Design review of the part built by this model. Coordinates are the model's own, in mm. Give positions to 0.01 mm unless a question says otherwise; leave off trailing zeros. Loops run counter-clockwise (first coordinate to the right, second up) from the corner with the lowest first, then second, coordinate; pieces in that order, holes last. Notation, with made-up numbers: M 57.25,-22.5 L 76.25,-22.5 A8 ccw 76.25,-15.5 Z; hole C 30,13 d4. An arc over 180 degrees is marked long. Use a Markdown table: item, result. Add a question column.
(1) Add section A-A, the plane y = 30. Give the boundary of the cut face in (x, z).
(2) Insertion check: pin 1 Ø3.5 at (x, y) = (115, 60) entering from +Z. The pin has a flat end and moves straight along its axis. Give the tip position at first contact, or say it passes through.
(3) For probe 1 along Y at (x, z) = (43, 0.75); probe 2 along X at (y, z) = (115, 0.9); probe 3 along X at (y, z) = (24.75, 0.8), list the stretches that pass through material, from the lowest coordinate up.
(4) Add section D-D, the plane x = 43. Give the boundary of the cut face in (y, z).
(5) Add section B-B, the plane x = 85. Give the boundary of the cut face in (y, z), then the cut area to 4 significant figures.
(6) Add section C-C, the plane y = 95.25. Give the boundary of the cut face in (x, z).
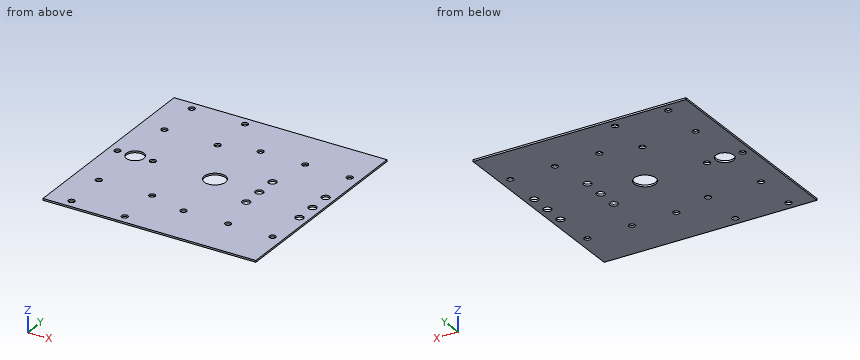
Autodesk Inventor part; units mm, degrees
ref_plane "作業平面1" through (0, 60, 0) normal (0, 1, 0) x (1, 0, 0)
ref_plane "YZ Plane" through (0, 0, 0) normal (1, 0, 0) x (0, 1, 0)
ref_plane "XZ Plane" through (0, 0, 0) normal (0, 1, 0) x (-1, 0, 0)
sketch "スケッチ1" plane through (0, 0, 0) normal (0, 0, 1) x (1, 0, 0)
  line L0 (0, 0) -> (120, 0)
  line L1 (120, 0) -> (120, 120)
  line L2 (120, 120) -> (0, 120)
  line L3 (0, 120) -> (0, 0)
  dimension "d0" = 120
  dimension "d1" = 120
extrude "押し出し1" add sketch "スケッチ1" along normal blind 1
sketch "スケッチ2" plane through (0, 0, 1) normal (0, 0, 1) x (1, 0, 0)
  line L0 (0, 120) -> (0, 0)
  line L1 (0, 60) -> (120, 60)
  line L2 (120, 0) -> (120, 120)
  circle A0 centre (60, 60) radius 6
  circle A1 centre (15, 60) radius 5
  circle A2 centre (115, 95.25) radius 1.5
  circle A3 centre (85, 95.25) radius 1.5
  line L3 (120, 120) -> (0, 120)
  circle A4 centre (5, 60) radius 1.75
  circle A5 centre (25, 60) radius 1.75
  dimension "d4" = 12
  dimension "d5" = 10
  dimension "d6" = 3
  dimension "d7" = 3
  dimension "d8" = 15
  dimension "d9" = 30
  dimension "d10" = 5
  dimension "d11" = 24.75
  dimension "d12" = 24.75
  dimension "d13" = 3.5
  dimension "d14" = 3.5
  dimension "d15" = 20
  dimension "d16" = 5
extrude "押し出し2" cut sketch "スケッチ2" against normal through all contours A4 L1 | L1 A4 | A0 L1 | L1 A0 | A1 L1 | L1 A1 | A5 L1 | L1 A5 | A2 | A3
sketch "スケッチ3" plane through (0, 0, 1) normal (0, 0, 1) x (1, 0, 0)
  line L0 (0, 120) -> (0, 0)
  line L1 (0, 60) -> (120, 60) construction
  line L2 (120, 0) -> (120, 120)
  line L3 (120, 120) -> (0, 120) construction
  point P0 (13, 115)
  point P1 (43, 115)
  point P2 (13, 90)
  point P3 (43, 90)
  point P4 (13, 5)
  point P5 (43, 5)
  point P6 (13, 30)
  point P7 (43, 30)
  dimension "d19" = 5
  dimension "d20" = 13
  dimension "d23" = 30
  dimension "d26" = 25
hole "穴1" at (13, 115, 1) at (43, 115, 1) at (13, 90, 1) at (43, 90, 1) at (13, 5, 1) at (43, 5, 1) at (43, 30, 1) at (13, 30, 1) direction (0, 0, -1) diameter 3.5 end through all
sketch "スケッチ4" plane through (0, 0, 1) normal (0, 0, 1) x (1, 0, 0)
  point P0 (0, 0)
sketch "スケッチ5" plane through (0, 0, 1) normal (0, 0, 1) x (1, 0, 0)
  circle A0 centre (85, 95.25) radius 1.5
  circle A1 centre (85, 95.25) radius 1.5
  circle A2 centre (115, 95.25) radius 1.5
  circle A3 centre (115, 95.25) radius 1.5
  point P0 (0, 0)
extrude "押し出し3" add sketch "スケッチ5" against normal blind 1
sketch "スケッチ6" plane through (0, 0, 1) normal (0, 0, 1) x (1, 0, 0)
  line L0 (0, 120) -> (0, 0)
  line L1 (0, 60) -> (120, 60) construction
  line L2 (120, 0) -> (120, 120)
  line L3 (0, 0) -> (120, 0)
  line L4 (50.2, 60) -> (170.2, 60) construction
  line L5 (120, 120) -> (0, 120)
  point P0 (64, 24.75)
  point P1 (114.2, 24.75)
  point P2 (85, 48)
  point P3 (115, 48)
  point P4 (64, 95.25)
  point P5 (114.2, 95.25)
  point P6 (85, 72)
  point P7 (115, 72)
  dimension "d38" = 64
  dimension "d39" = 24.75
  dimension "d42" = 50.2
  dimension "d47" = 72
  dimension "d48" = 85
  dimension "d51" = 30
hole "穴2" at (64, 24.75, 1) at (114.2, 24.75, 1) at (85, 48, 1) at (115, 48, 1) at (85, 72, 1) at (115, 72, 1) at (64, 95.25, 1) at (114.2, 95.25, 1) direction (0, 0, -1) diameter 3.5 end through all
sketch "スケッチ7" plane through (0, 0, 1) normal (0, 0, 1) x (1, 0, 0)
  circle A0 centre (85, 72) radius 1.75
  circle A1 centre (85, 72) radius 2.25
  circle A2 centre (115, 72) radius 1.75
  circle A3 centre (115, 72) radius 2.25
  circle A4 centre (115, 48) radius 1.75
  circle A5 centre (115, 48) radius 2.25
  circle A6 centre (85, 48) radius 1.75
  circle A7 centre (85, 48) radius 2.25
  point P0 (0, 0)
  dimension "d63" = 4.5
  dimension "d64" = 4.5
  dimension "d65" = 4.5
  dimension "d66" = 4.5
extrude "押し出し4" cut sketch "スケッチ7" against normal blind 1 contours A0 | A1 | A2 | A3 | A4 | A5 | A6 | A7
sketch "スケッチ9" plane through (0, 0, 1) normal (0, 0, 1) x (1, 0, 0)
  circle A0 centre (85, 72) radius 2.25 construction
  circle A1 centre (85, 48) radius 2.25 construction
  line L0 (85, 72) -> (85, 48) construction
  circle A2 centre (115, 72) radius 2.25 construction
  circle A3 centre (115, 48) radius 2.25 construction
  line L1 (115, 72) -> (115, 48) construction
  point P0 (0, 0)
  point P1 (85, 60)
  point P2 (115, 60)
hole "穴3" at (85, 60, 1) at (115, 60, 1) direction (0, 0, -1) diameter 4.5 depth 1
ref_plane "作業平面1" through (0, 60, 0) normal (0, 1, 0) x (1, 0, 0)
sketch "スケッチ10" plane through (0, 0, 1) normal (0, 0, 1) x (1, 0, 0)
  circle A0 centre (64, 95.25) radius 1.75
  circle A1 centre (114.2, 95.25) radius 1.75
  line L0 (64, 95.25) -> (114.2, 95.25)
  circle A2 centre (85, 60) radius 2.25
  circle A3 centre (115, 60) radius 2.25
  line L1 (85, 60) -> (115, 60)
  point P0 (0, 0)
  point P1 (89.1, 95.25)
  point P2 (89.1, 24.75)
hole "穴4" at (89.1, 95.25, 1) at (89.1, 24.75, 1) direction (0, 0, -1) diameter 3.4 depth 1
properties part number "RD002_フレーム" material "アルミニウム 6061"
Established:
| question | item | result |
|---|---|---|
| 1 | outline | M 0,0 L 11.25,0 L 11.25,1 L 0,1 Z; M 14.75,0 L 41.25,0 L 41.25,1 L 14.75,1 Z; M 44.75,0 L 120,0 L 120,1 L 44.75,1 Z |
| 2 | pin 1 | through |
| 3 | probe 1 | 0 to 3.25, 6.75 to 28.25, 31.75 to 88.25, 91.75 to 113.25, 116.75 to 120 |
| 3 | probe 2 | 0 to 11.25, 14.75 to 41.25, 44.75 to 120 |
| 3 | probe 3 | 0 to 62.25, 65.75 to 87.4, 90.8 to 112.45, 115.95 to 120 |
| 4 | outline | M 0,0 L 3.25,0 L 3.25,1 L 0,1 Z; M 6.75,0 L 28.25,0 L 28.25,1 L 6.75,1 Z; M 31.75,0 L 88.25,0 L 88.25,1 L 31.75,1 Z; M 91.75,0 L 113.25,0 L 113.25,1 L 91.75,1 Z; M 116.75,0 L 120,0 L 120,1 L 116.75,1 Z |
| 5 | outline | M 0,0 L 45.75,0 L 45.75,1 L 0,1 Z; M 50.25,0 L 57.75,0 L 57.75,1 L 50.25,1 Z; M 62.25,0 L 69.75,0 L 69.75,1 L 62.25,1 Z; M 74.25,0 L 120,0 L 120,1 L 74.25,1 Z |
| 5 | area | 106.5 mm^2 |
| 6 | outline | M 0,0 L 62.25,0 L 62.25,1 L 0,1 Z; M 65.75,0 L 87.4,0 L 87.4,1 L 65.75,1 Z; M 90.8,0 L 112.45,0 L 112.45,1 L 90.8,1 Z; M 115.95,0 L 120,0 L 120,1 L 115.95,1 Z |
